Check sheet for the drawn part. Datum: minimum x, y, z corner. Units: mm. A direction names the side the tool comes from. Coordinates: 2 decimals unless noted, no trailing zeros. Order: outer loops, then holes, each group sorted by start corner. A loop starts at its lowest first (then second) coordinate and runs counter-clockwise, first axis right, second up. Notation, with made-up numbers: (26.5, 23) - (35.5, 23) arc R24 ccw to (35.5, 45) - close; hole circle Ø3 at (86.25, 25). An arc over 180 degrees is marked (long way). Put each result on its own line as item: value.
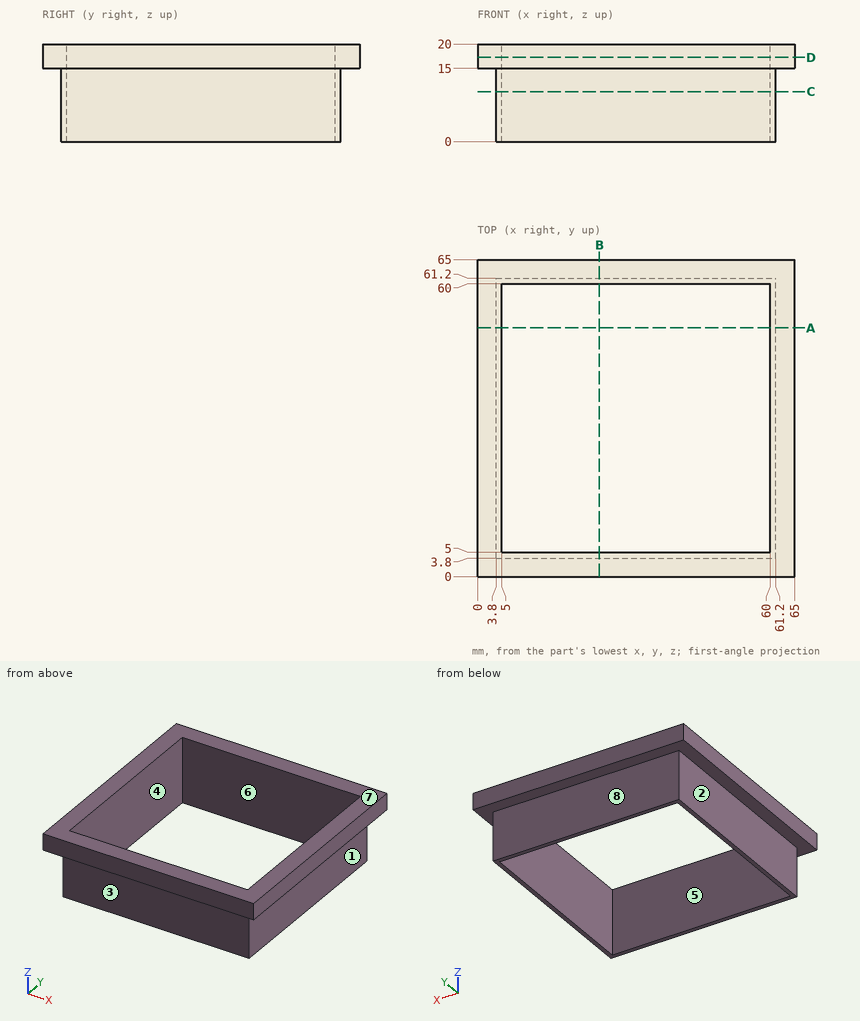
Q1. Access from +Z, -Z, +X, -X, +Y, -Y to the whole of each face (thin tool, end or side, straight path). Record for the marked faces 1, 2, 3 and 4.
Answer block:
face 1: -Z, +X, +Y, -Y
face 2: -Z, -X, +Y, -Y
face 3: -Z, +X, -X, -Y
face 4: +Z, -Z
Q2. Section check A-A on y = 51. Record the boundary of the cut face in (x, z).
Answer block:
outline: (0, 15) - (3.8, 15) - (3.8, 0) - (5, 0) - (5, 20) - (0, 20) - close; (60, 0) - (61.2, 0) - (61.2, 15) - (65, 15) - (65, 20) - (60, 20) - close
Q3. Draft check along Y on the marked faces 5, 6, 7 and 8. Enter one of: pulls with the +Y half, pulls with the -Y half, needs draft (parallel to the pull), parting line crosses it, or undercut.
Answer block:
face 5: undercut
face 6: undercut
face 7: needs draft
face 8: pulls with the +Y half
Q4. Section check D-D on z = 17.25. Record the boundary of the cut face in (x, y).
Answer block:
outline: (0, 0) - (65, 0) - (65, 65) - (0, 65) - close; hole (5, 5) - (60, 5) - (60, 60) - (5, 60) - close
Q5. Thickness scan on L1, parallel to Y at x = 50.5, z = 13; L2, parallel to Y at x = 55, z = 19.25. Record the ranges inside material, lowest first. Write a range as [from, to].
Answer block:
L1: y = [3.8, 5], [60, 61.2]
L2: y = [0, 5], [60, 65]
Q6. Depth check by flat-ended pin: pin 1 Ø4.5 at (y, z) = (26, 6.5) entering from +X; pin 2 Ø12 at (y, z) = (31.5, 4) entering from -X; pin 3 Ø4.5 at (x, z) = (41, 9.5) entering from -Y; pin 4 Ø10 at (y, z) = (49.5, 10.5) entering from -X. Enter the tip coordinate at first touch or a pass-through.
Answer block:
pin 1: stops at x = 61.2
pin 2: stops at x = 3.8
pin 3: stops at y = 3.8
pin 4: stops at x = 0
Q7. Section check C-C on z = 10.25. Record the boundary of the cut face in (x, y).
Answer block:
outline: (3.8, 3.8) - (61.2, 3.8) - (61.2, 61.2) - (3.8, 61.2) - close; hole (5, 5) - (60, 5) - (60, 60) - (5, 60) - close
